Geometry: see drawing. Coordinates: mm, zero at the bounding-box minimum. Round coordinates to 2 decimals unless told otherwise and drop trailing zeros. Loops run counter-clockwise (first coordinate to the right, second up) from the corner with the lowest first, then second, coordinate; pieces in that order, holes last. Notation, with made-up numbers: (89.25, -14.75) -> (103.25, -14.75) arc R19 ccw to (103.25, 4.25) -> close; hole circle Ø8 at (66, -5.5). An arc over 180 degrees is marked (long way). Write item = value, one per line.
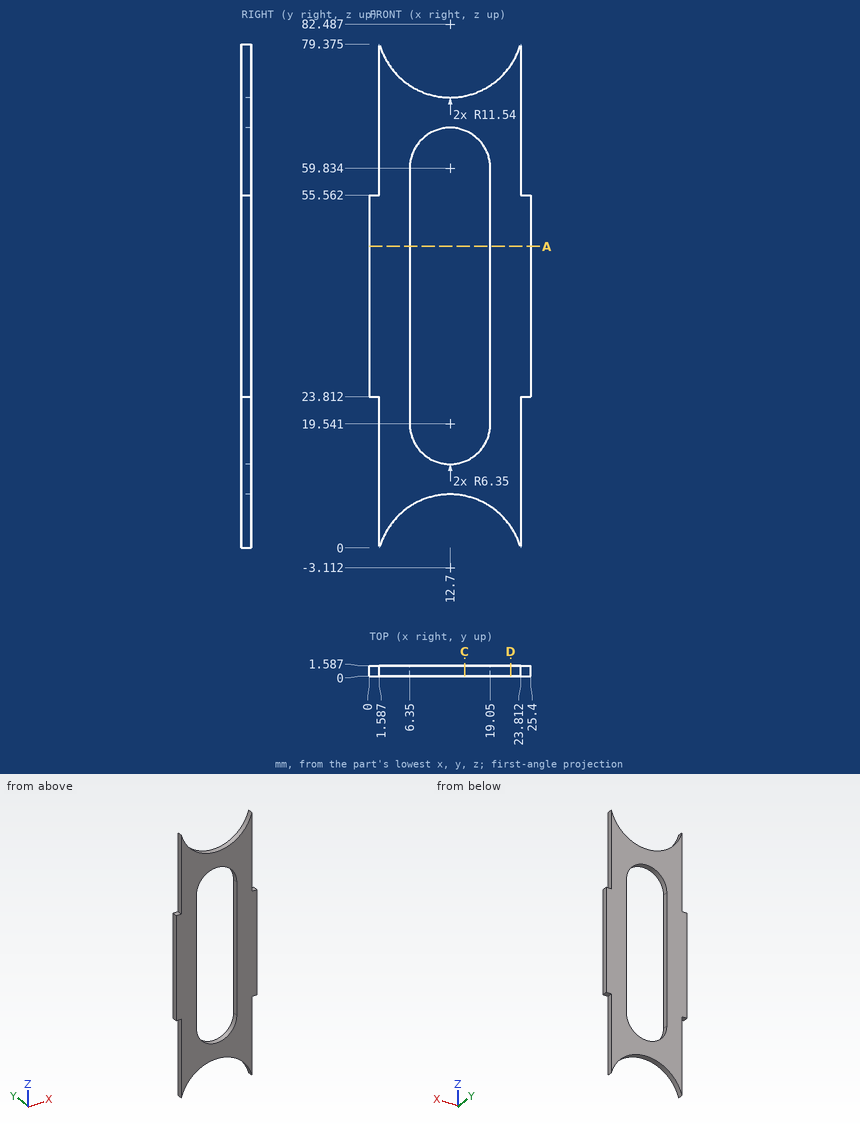
1. Section query D-D (x = 22.25). Return the cut outline in (y, z), then the cut area to 3 significant figures.
Evaluation:
outline = (0, 3.37) -> (1.59, 3.37) -> (1.59, 76.01) -> (0, 76.01) -> close
area = 115 mm²
2. Line query: probe 1 along X at (y, z) = (0.65, 52.5); probe 2 along Z at (x, y) = (12.25, 0.7) (1 decimal); probe 3 along X at (y, z) = (0.1, 20.5). Output: solid intervals per line, ascending. Write a range as from..to.
Evaluation:
probe_1 = 0..6.35, 19.05..25.4
probe_2 = 8.4..13.2, 66.2..71
probe_3 = 1.59..6.35, 19.05..23.81
3. Section query A-A (z = 47.5). Return the cut outline in (x, y).
Evaluation:
outline = (0, 0) -> (6.35, 0) -> (6.35, 1.59) -> (0, 1.59) -> close; (19.05, 0) -> (25.4, 0) -> (25.4, 1.59) -> (19.05, 1.59) -> close
4. Contact query for flat-ended pins moving along their axis: pin 1 Ø0.5 at (y, z) = (1, 62.5) entering from +X; pin 2 Ø0.8 at (y, z) = (0.5, 14) entering from -X; pin 3 Ø0.5 at (x, y) = (25, 0.5) entering from +Z. Output: stop coordinate, or through.
Evaluation:
pin_1 = 23.81
pin_2 = 1.59
pin_3 = 55.56
5. Section query C-C (x = 15). Return the cut outline in (y, z).
Evaluation:
outline = (0, 8.2) -> (1.59, 8.2) -> (1.59, 13.62) -> (0, 13.62) -> close; (0, 65.75) -> (1.59, 65.75) -> (1.59, 71.18) -> (0, 71.18) -> close
